```python
from build123d import *

# Parameters (mm, degrees)
FILLET1_R          = 2
CUT_EXTRUDE1_DEPTH = 7
CUT_EXTRUDE2_DEPTH = 8.42


with BuildPart() as part:
    # Sketch1 → Revolve1 (revolve)
    with BuildSketch(Plane.XY, mode=Mode.PRIVATE) as revolve1_sk:
        Polygon((-305.228973115, 0), (-305.228973115, 37.5), (-266.228973115, 37.5), (-266.228973115, 42.5), (-251.228973115, 42.5), (-251.228973115, 55), (-228.728973115, 55), (-228.728973115, 45), (-103.728973115, 45), (-103.728973115, 42.5), (33.771026885, 42.5), (33.771026885, 37.5), (70.771026885, 37.5), (70.771026885, 35), (140.771026885, 35), (140.771026885, 32.5), (230.771026885, 32.5), (230.771026885, 0), align=None)
    revolve(revolve1_sk.sketch.rotate(Axis((-305.228973115, 0, 0), (1, 0, 0)), 90), axis=Axis((-305.228973115, 0, 0), (1, 0, 0)))

    # Fillet1
    fillet1_edges = [part.edges().sort_by_distance(p)[0] for p in [
        (230.771026885, 0, -32.5),
        (-305.228973115, 0, -37.5),
    ]]
    fillet(fillet1_edges, radius=FILLET1_R)

    # Sketch2 → Cut-Extrude1 (cut)
    with BuildSketch(Plane(origin=(0, 45, 0), x_dir=(1, 0, 0), z_dir=(0, 1, 0))):
        with BuildLine():
            Line((-214.728973115, 9), (-117.728973115, 9))
            ThreePointArc((-117.728973115, 9), (-108.728973115, 0), (-117.728973115, -9))
            Line((-117.728973115, -9), (-214.728973115, -9))
            ThreePointArc((-214.728973115, -9), (-223.728973115, 0), (-214.728973115, 9))
        make_face()
    extrude(amount=-CUT_EXTRUDE1_DEPTH, mode=Mode.SUBTRACT)

    # Sketch3 → Cut-Extrude2 (cut)
    with BuildSketch(Plane(origin=(0, 32.5, 0), x_dir=(1, 0, 0), z_dir=(0, 1, 0))):
        with BuildLine():
            Line((160.771026885, 8), (239.672202356, 8))
            ThreePointArc((239.672202356, 8), (247.672202356, 0), (239.672202356, -8))
            Line((239.672202356, -8), (160.771026885, -8))
            ThreePointArc((160.771026885, -8), (152.771026885, 0), (160.771026885, 8))
        make_face()
    extrude(amount=-CUT_EXTRUDE2_DEPTH, mode=Mode.SUBTRACT)


solid = part.part
```
CAD build for the part. Positions are in the model's coordinates, mm. A direction names the side the tool comes from. Round coordinates to 2 decimals unless told otherwise and drop trailing zeros. Order: outer loops, then holes, each group sorted by start corner. A loop starts at its lowest first (then second) coordinate and runs counter-clockwise, first axis right, second up. Notation, with made-up numbers: (5, -12.5) - (50, -12.5) arc R4 cw to (50, -6.5) - close; hole circle Ø3 at (-38.75, 50.25). An arc over 180 degrees is marked (long way). Use CSV: the item, a comma, the result in double quotes. Start each with the question number.
1) Saw through at A-A (x = 167.5). List the corners of the cut face in (y, z).
2) Saw through at C-C (x = -64). List the corners of the cut face in (y, z), and give its area (3 significant figures).
3) Wall check: L1, parallel to Y at x = -232, z = 3; L2, parallel to X at y = -15, z = 48; L3, parallel to X at y = -25, z = -25.5. Give the ranges that are in metal, low to high. Write a range as [from, to].
4) Pin check, flat tips, straight feed: pin 1 Ø3 at (x, z) = (-200, 37.5) entering from -Y; pin 2 Ø6 at (x, y) = (29, -19) entering from -Z; pin 3 Ø5 at (x, y) = (-186.5, 41) entering from -Z. Stop position of each tip, or through.
5) Tool access for faces 1 (the flat face through (33.771, 38, 0)), 2 (the cylindrical face through (-108.73, 41.55, -0.2)), 3 (the cylindrical face through (152.773, 28.349, 0.176)), 4 (the flat face through (-266.229, 38, 0)), 5 (the cylindrical face through (-239.821, 48.794, 25.379)): list every direction of +Z, -Z, +X, -X, +Y, -Y with a clear straight run to the whole face (end or side of a thin tool).
6) Saw through at B-B (x = 96.5). List the corners of the cut face in (y, z), and give its area (3 significant figures).
7) Two-plate mould, pull along X, no slides. Class faces 6 (the cylindrical face through (-284.47, 33.27, 17.3)), 7 (the flat face through (-305.229, 0, 0)), 8 (the cylindrical face through (-223.727, 41.549, 0.198)), 9 (the flat face through (-165, 38, 0)): pulls with the +X half, pulls with the -X half, needs draft (parallel to the pull), parting line crosses it, or undercut.
Values follow:
1,outline,"(24.08, -8) - (24.08, 8) - (31.5, 8) arc R32.5 ccw (long way) to (31.5, -8) - close"
2,outline,"circle Ø85 at (0, 0)"
2,area,"5,670 mm2"
3,L1,"y = [-54.92, 54.92]"
3,L2,"x = [-251.23, -228.73]"
3,L3,"x = [-305.22, 70.77]"
4,pin 1,"stops at y = -27"
4,pin 2,"stops at z = -39.37"
4,pin 3,"stops at z = -23.3"
5,face 1,"+X"
5,face 2,"+Y"
5,face 3,"+X, +Y"
5,face 4,"-X"
5,face 5,"+X, -X"
6,outline,"circle Ø70 at (0, 0)"
6,area,"3,850 mm2"
7,face 6,"needs draft"
7,face 7,"pulls with the -X half"
7,face 8,"undercut"
7,face 9,"undercut"
